Input: part model. Units: mm. Frame: model coordinates. A direction names the side the tool comes from. Coordinates: 2 decimals unless noted, no trailing zeros. Loops run counter-clockwise (first coordinate to the right, second up) from the corner with the lowest first, then second, coordinate; pieces in that order, holes last. Notation, with made-up numbers: M 22.5,12 L 67.5,12 A26 ccw 67.5,51 Z; hole C 10.5,64 d3. An arc over 180 degrees is marked long. Use a Markdown table: item, result. Add a question column.
1. Section C-C on z = 0. Output: boundary loops of the cut face in (x, y).
2. Section A-A on y = 5.25. Output: boundary loops of the cut face in (x, z), then the cut area to 3 significant figures.
3. Line query: L1, parallel to X at y = 4, z = 0; L2, parallel to X at y = 8.75, z = 2.75; L3, parallel to X at y = 7.5, z = 0.25. Output: solid intervals per line, ascending. Write a range as [from, to].
4. Draft query along Z for faces 3 (the cylindrical face through (-10, 4, 0)), 4 (the flat face through (0, 5, 0)), 5 (the flat face through (0, 3, -5)), 6 (the flat face through (0, 3, 5)). Return one class per face: +Z half, -Z half, draft (parallel to the pull), parting line (faces both ways), or undercut.
5. Section B-B on x = 8.5. Output: boundary loops of the cut face in (y, z), then the cut area to 3 significant figures.
6. Set-up query: faces 1 (the flat face through (-10, 9, -1)), 2 (the flat face through (6, 7, 0)). Return all of +Z, -Z, +X, -X, +Y, -Y with unobstructed straight access to the full face (end or side cutting, diameter ignored); none if empty.
7. Section D-D on z = -3. Output: boundary loops of the cut face in (x, y).
8. Pin query (flat end, axial travel): pin 1 (1.5 mm diameter, centred on x = -4.5, z = 2.5, fed in from +Y). Return the tip coordinate at first contact, or that it passes through.
```python
from build123d import *

# Parameters (mm, degrees)
SKETCH_1_W      = 22
SKETCH_1_H      = 10
SKETCH_1_R      = 1.5
EXTRUDE_1_DEPTH = 5
SKETCH_2_W      = 5
SKETCH_2_H      = 10
SKETCH_2_R      = 1.5
EXTRUDE_2_DEPTH = 4


with BuildPart() as part:
    # 草圖1 → 填料-伸長1 (new body)
    with BuildSketch(Plane(origin=(0, 0, 0), x_dir=(1, 0, 0), z_dir=(0, 1, 0))):
        Rectangle(SKETCH_1_W, SKETCH_1_H)
        with Locations((-8.5, 0)):
            Circle(SKETCH_1_R, mode=Mode.SUBTRACT)
        with Locations((8.5, 0)):
            Circle(SKETCH_1_R, mode=Mode.SUBTRACT)
    extrude(amount=EXTRUDE_1_DEPTH)

    # 草圖2 → 填料-伸長2 (add)
    with BuildSketch(Plane(origin=(0, 5, 0), x_dir=(1, 0, 0), z_dir=(0, 1, 0))):
        with Locations((-8.5, 0)):
            Rectangle(SKETCH_2_W, SKETCH_2_H)
        with Locations((-8.5, 0)):
            Circle(SKETCH_2_R, mode=Mode.SUBTRACT)
        with Locations((8.5, 0)):
            Rectangle(SKETCH_2_W, SKETCH_2_H)
        with Locations((8.5, 0)):
            Circle(SKETCH_2_R, mode=Mode.SUBTRACT)
    extrude(amount=EXTRUDE_2_DEPTH)


solid = part.part
```
Answers below:
| question | item | result |
|---|---|---|
| 1 | outline | M -11,0 L -10,0 L -10,9 L -11,9 Z; M -7,0 L 7,0 L 7,9 L 6,9 L 6,5 L -6,5 L -6,9 L -7,9 Z; M 10,0 L 11,0 L 11,9 L 10,9 Z |
| 2 | outline | M -11,-5 L -6,-5 L -6,5 L -11,5 Z; M 6,-5 L 11,-5 L 11,5 L 6,5 Z; hole C -8.5,0 d3; hole C 8.5,0 d3 |
| 2 | area | 85.9 mm² |
| 3 | L1 | x = [-11, -10], [-7, 7], [10, 11] |
| 3 | L2 | x = [-11, -6], [6, 11] |
| 3 | L3 | x = [-11, -9.98], [-7.02, -6], [6, 7.02], [9.98, 11] |
| 4 | face 3 | undercut |
| 4 | face 4 | draft |
| 4 | face 5 | -Z half |
| 4 | face 6 | +Z half |
| 5 | outline | M 0,-5 L 9,-5 L 9,-1.5 L 0,-1.5 Z; M 0,1.5 L 9,1.5 L 9,5 L 0,5 Z |
| 5 | area | 63.0 mm² |
| 6 | face 1 | +Z, -Z, +X, -X, +Y |
| 6 | face 2 | +Z, -Z, +Y |
| 7 | outline | M -11,0 L 11,0 L 11,9 L 6,9 L 6,5 L -6,5 L -6,9 L -11,9 Z |
| 8 | pin 1 | stops at y = 5 |
